Autodesk Fusion 360 part; units mm, degrees
sketch "スケッチ1" plane through (0, 0, 0) normal (0, 1, 0) x (1, 0, 0)
  line L0 (0, 8) -> (0, -10)
  line L1 (-10, 0) -> (10, 0)
  line L2 (-6.5, 6.5) -> (6.5, 6.5)
  line L3 (6.5, 6.5) -> (6.5, -6.5)
  line L4 (6.5, -6.5) -> (-6.5, -6.5)
  line L5 (-6.5, -6.5) -> (-6.5, 6.5)
  line L6 (-5, 5) -> (5, 5)
  line L7 (5, 5) -> (5, -5)
  line L8 (5, -5) -> (-5, -5)
  line L9 (-5, -5) -> (-5, 5)
  dimension "d1" = 13
  dimension "d2" = 13
extrude "押し出し1" add sketch "スケッチ1" along normal blind 13 contours L0 L1 L2 L3 L6 L7 | L0 L1 L2 L5 L6 L9 | L0 L1 L4 L5 L8 L9 | L0 L1 L3 L4 L7 L8
sketch "スケッチ2" plane through (0, 0, 6.5) normal (0, 0, 1) x (1, 0, 0)
  line L0 (-6.5, 0) -> (6.5, 0)
  line L1 (6.5, 0) -> (6.5, 13)
  line L2 (6.5, 13) -> (-6.5, 13)
  line L3 (-6.5, 13) -> (-6.5, 0)
  point P0 (0, 6.5)
  dimension "d5" = 6.5
  dimension "d6" = 6.5
hole "穴1" at (0, 6.5, 6.5) direction (0, 0, -1) diameter 3.2 depth 20 tip angle 118
sketch "スケッチ3" plane through (6.5, 0, 0) normal (1, 0, 0) x (0, 0, -1)
  line L0 (-6.5, 0) -> (6.5, 0)
  line L1 (6.5, 0) -> (6.5, 13)
  line L2 (6.5, 13) -> (-6.5, 13)
  line L3 (-6.5, 13) -> (-6.5, 0)
  line L4 (-9, 6.5) -> (10, 6.5)
  line L5 (0, 14) -> (0, -2)
  line L6 (-5, 11.5) -> (5, 11.5)
  line L7 (5, 11.5) -> (5, 1.5)
  line L8 (5, 1.5) -> (-5, 1.5)
  line L9 (-5, 1.5) -> (-5, 11.5)
  dimension "d10" = 10
  dimension "d11" = 10
extrude "押し出し2" cut sketch "スケッチ3" against normal blind 17 contours L4 L5 L8 L9 | L4 L5 L7 L8 | L4 L5 L6 L9 | L4 L5 L6 L7
extrude "押し出し3" add 1 faces at (6.5, 4.8333, -6) along direction (1, 0, 0) blind 13
extrude "押し出し4" add 1 faces at (-6.5, 4.8333, 6) along direction (-1, 0, 0) blind 13
sketch "スケッチ4" plane through (0, 13, 0) normal (0, 1, 0) x (-1, 0, 0)
  line L0 (-5, 5) -> (5, 5)
  line L1 (5, 5) -> (5, -5)
  line L2 (5, -5) -> (-5, -5)
  line L3 (-5, -5) -> (-5, 5)
  line L4 (19.5, 6.5) -> (-19.5, 6.5)
  line L5 (-19.5, 6.5) -> (-19.5, -6.5)
  line L6 (-19.5, -6.5) -> (19.5, -6.5)
  line L7 (19.5, -6.5) -> (19.5, 6.5)
sketch "スケッチ5" plane through (0, 0, -6.5) normal (0, 0, -1) x (-1, 0, 0)
  circle A0 centre (0, 6.5) radius 1.6
  line L0 (-19.5, 0) -> (19.5, 0)
  line L1 (19.5, 0) -> (19.5, 13)
  line L2 (19.5, 13) -> (-19.5, 13)
  line L3 (-19.5, 13) -> (-19.5, 0)
  line L4 (-19.5, 13) -> (19.5, 13)
  point P0 (-13, 6.5)
  point P1 (13, 6.5)
  dimension "d18" = 6.5
  dimension "d19" = 6.5
  dimension "d20" = 6.5
  dimension "d21" = 6.5
hole "穴2" at (13, 6.5, -6.5) at (-13, 6.5, -6.5) direction (0, 0, 1) diameter 3.2 depth 100 tip angle 118
extrude "押し出し5" cut 1 faces at (19.5, 4.8333, -6) along direction (-1, 0, 0) blind 2
extrude "押し出し6" cut 1 faces at (-19.5, 4.8333, 6) along direction (1, 0, 0) blind 2
sketch "スケッチ6" plane through (0, 0, 6.5) normal (0, 0, 1) x (1, 0, 0)
  line L0 (-17.5, 13) -> (-17.5, 0)
  line L1 (-17.5, 0) -> (17.5, 0)
  line L2 (17.5, 0) -> (17.5, 13)
  line L3 (17.5, 13) -> (-17.5, 13)
  circle A0 centre (0, 6.5) radius 1.6
  circle A1 centre (-13, 6.5) radius 1.6
  circle A2 centre (13, 6.5) radius 1.6
  line L4 (-13, 6.5) -> (-9.8, 6.5)
  circle A3 centre (-9.8, 6.5) radius 1.6
  line L5 (13, 6.5) -> (9.8, 6.5)
  circle A4 centre (9.8, 6.5) radius 1.6
  line L6 (-9.8, 6.5) -> (-6.6, 6.5)
  line L7 (9.8, 6.5) -> (6.6, 6.5)
  circle A5 centre (-6.6, 6.5) radius 1.6
  circle A6 centre (6.6, 6.5) radius 1.6
  line L8 (-13, 6.5) -> (-13, 8.1)
  line L9 (-13, 6.5) -> (-13, 4.9)
  line L10 (-13, 8.1) -> (-6.6, 8.1)
  line L11 (-13, 4.9) -> (-6.6, 4.9)
  line L12 (13, 6.5) -> (13, 8.1)
  line L13 (13, 6.5) -> (13, 4.9)
  line L14 (13, 8.1) -> (6.6, 8.1)
  line L15 (13, 4.9) -> (6.6, 4.9)
  dimension "d29" = 3.2
  dimension "d30" = 3.2
  dimension "d31" = 3.2
  dimension "d32" = 3.2
extrude "押し出し7" cut sketch "スケッチ6" against normal blind 13 contours A1 A3 L11 | L4 A3 L6 | A1 A3 L10 | L4 A3 L6 | A3 A5 L10 | A3 A5 L11 | A5 | A2 A4 L14 | A2 A4 L15 | L5 A4 L7 | L5 A4 L7 | A4 A6 L14 | A4 A6 L15 | A6
Can you work these out from the model? Positions are in its coordinate system, mm. A direction names the side the tool comes from. Coordinates: 2 decimals unless noted, no trailing zeros. Loops run counter-clockwise (first coordinate to the right, second up) from the corner with the lowest first, then second, coordinate; pieces in that order, holes last.
1) Thinking about a two-plate mould opening in Y: for faces 6 (the flat face through (0, 0, 6)), 7 (the flat face through (17.5, 6, -6)), 8 (the cylindrical face through (-14.6, 6.5, 5.8)), which applies, pulls with the +Y half, pulls with the -Y half, needs draft (parallel to the pull), parting line crosses it, or undercut?
2) I need wall thicknesses on probe 1 along X at (y, z) = (6.5, -6.1); probe 2 along Z at (x, y) = (-4, 2.5); probe 3 along Y at (x, z) = (0, -5.4). Which ranges of each line are inside material? Lowest first, please.
3) Imagine slicing it at A-A on y = 3.75. List the corners of the cut face in (x, z) for me.
4) Imagine slicing it at D-D on y = 7.5. State how many separate pieces and enclosed holes the cut face has, plus the area to 3 significant figures.
5) Imagine slicing it at B-B on x = 8.5. List the corners of the cut face in (y, z) for me, plus the area to 3 significant figures.
6) Which directions (+Z, -Z, +X, -X, +Y, -Y) give clear straight access to the entire face, cutting with the end or side of a thin tool? Please do faces 1 (the flat face through (-17.5, 6, 6)), 2 (the flat face through (-10, 8.1, -6)), 3 (the flat face through (-5, 12, 0)), 4 (the flat face through (11, 1.5, 0)), 5 (the flat face through (0, 4, 6.5)).
7) Imagine slicing it at C-C on z = -0.25. List the corners of the cut face in (x, y) for me, plus the area to 3 significant figures.
Completed:
1. face 6: pulls with the -Y half
1. face 7: needs draft
1. face 8: undercut
2. probe 1: x = -17.5 to -14.6, -5 to -1.6, 1.6 to 5, 14.6 to 17.5
2. probe 2: z = -6.5 to -5, 5 to 6.5
2. probe 3: y = 0 to 4.9, 8.1 to 13
3. outline: (-17.5, -6.5) - (17.5, -6.5) - (17.5, -5) - (-17.5, -5) - close; (-17.5, 5) - (17.5, 5) - (17.5, 6.5) - (-17.5, 6.5) - close
4. separate pieces: 8
4. enclosed holes: 0
4. area: 44.1 mm2
5. outline: (0, -6.5) - (4.9, -6.5) - (4.9, -5) - (1.5, -5) - (1.5, 5) - (4.9, 5) - (4.9, 6.5) - (0, 6.5) - close; (8.1, -6.5) - (13, -6.5) - (13, 6.5) - (8.1, 6.5) - (8.1, 5) - (11.5, 5) - (11.5, -5) - (8.1, -5) - close
5. area: 59.4 mm2
6. face 1: +Z, -Z, -X, +Y, -Y
6. face 2: +Z, -Z
6. face 3: +Y, -Y
6. face 4: +X, -X
6. face 5: +Z, +X, -X, +Y, -Y
7. outline: (-17.5, 0) - (-5, 0) - (-5, 1.5) - (-17.5, 1.5) - close; (-17.5, 11.5) - (-5, 11.5) - (-5, 13) - (-17.5, 13) - close; (5, 0) - (17.5, 0) - (17.5, 1.5) - (5, 1.5) - close; (5, 11.5) - (17.5, 11.5) - (17.5, 13) - (5, 13) - close
7. area: 75.0 mm2
